Geometry: final body of the model. Coordinates: model frame, mm. Round coordinates to 2 decimals unless told otherwise and drop trailing zeros. Loops run counter-clockwise (first coordinate to the right, second up) from the corner with the lowest first, then second, coordinate; pieces in that order, holes last. Notation, with made-up numbers: (88, 22.5) - (139, 22.5) arc R19 ccw to (139, 46.5) - close; hole circle Ø7 at (54, 79.25). An arc over 180 degrees is marked (long way). Return JSON: item names as keys, results as strings. Group by question number.
1. Section A-A on x = -28. Return loops of the section in (y, z).
2. First-contact query: pin 1 Ø2 at (y, z) = (0, 0) entering from -X; pin 2 Ø3 at (x, z) = (8, -2) entering from -Y; pin 3 Ø1.5 at (x, y) = (-24, -2) entering from -Z; pin 4 Ø3.5 at (y, z) = (0, 0) entering from -X. Flat tips, straight axial feed; report the tip coordinate or a pass-through.
3. Material intervals for probe 1 along Y at (x, z) = (48.05, 0); probe 2 along Y at (x, z) = (-43, 0); probe 3 along Z at (x, y) = (-44.5, 0.5), sorted ascending.
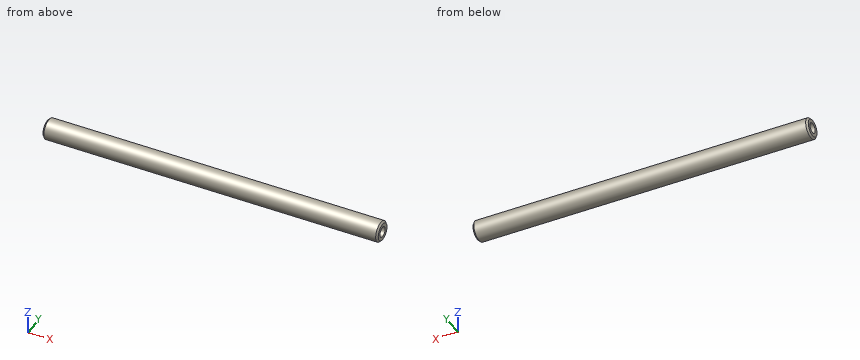
from build123d import *

# Parameters (mm, degrees)
SKETCH_1_W                     = 99
SKETCH_1_H                     = 3
CHAMFER_1_SIZE                 = 0.5
M3X0_5_1_D                     = 2.5
M3X0_5_1_DEPTH                 = 8.5
M3X0_5_1_CBORE_D               = 3
M3X0_5_1_CBORE_DEPTH           = 6
M3X0_5_1_TIP                   = 0.751075774
M3X0_5_1_ON_FACE_2_D           = 2.5
M3X0_5_1_ON_FACE_2_DEPTH       = 8.5
M3X0_5_1_ON_FACE_2_CBORE_D     = 3
M3X0_5_1_ON_FACE_2_CBORE_DEPTH = 6
M3X0_5_1_ON_FACE_2_TIP         = 0.751075774


with BuildPart() as part:
    # ｽｹｯﾁ1 → 回転1 (revolve)
    with BuildSketch(Plane.XY, mode=Mode.PRIVATE) as revolve_1_sk:
        with Locations((0, 1.5)):
            Rectangle(SKETCH_1_W, SKETCH_1_H)
    revolve(revolve_1_sk.sketch.rotate(Axis((0, 0, 0), (1, 0, 0)), 90), axis=Axis((0, 0, 0), (1, 0, 0)))

    # 面取り1
    chamfer_1_edges = [part.edges().sort_by_distance(p)[0] for p in [
        (49.5, 0, -3),
        (-49.5, 0, -3),
    ]]
    chamfer(chamfer_1_edges, length=CHAMFER_1_SIZE)

    # M3x0.5 ねじ穴1
    with Locations(Plane(origin=(49.5, 0, 0), x_dir=(0, 0, 1), z_dir=(1, 0, 0))):
        with Locations((0, 0)):
            CounterBoreHole(M3X0_5_1_D / 2, M3X0_5_1_CBORE_D / 2, M3X0_5_1_CBORE_DEPTH, depth=M3X0_5_1_DEPTH)
            with Locations((0, 0, -(M3X0_5_1_DEPTH + M3X0_5_1_TIP / 2))):  # 118° drill point
                Cone(0, M3X0_5_1_D / 2, M3X0_5_1_TIP, mode=Mode.SUBTRACT)

    # M3x0.5 ねじ穴1 on face 2
    with Locations(Plane(origin=(-49.5, 0, 0), x_dir=(0, 0, -1), z_dir=(-1, 0, 0))):
        with Locations((0, 0)):
            CounterBoreHole(M3X0_5_1_ON_FACE_2_D / 2, M3X0_5_1_ON_FACE_2_CBORE_D / 2, M3X0_5_1_ON_FACE_2_CBORE_DEPTH, depth=M3X0_5_1_ON_FACE_2_DEPTH)
            with Locations((0, 0, -(M3X0_5_1_ON_FACE_2_DEPTH + M3X0_5_1_ON_FACE_2_TIP / 2))):  # 118° drill point
                Cone(0, M3X0_5_1_ON_FACE_2_D / 2, M3X0_5_1_ON_FACE_2_TIP, mode=Mode.SUBTRACT)


solid = part.part
Taken from the geometry:
{
 "1": {"outline": "circle Ø6 at (0, 0)"},
 "2": {"pin 1": "x = -40.85", "pin 2": "y = -2.96", "pin 3": "z = -2.73", "pin 4": "x = -49.5"},
 "3": {"probe 1": "-3 to -1.5, 1.5 to 3", "probe 2": "-3 to -1.25, 1.25 to 3", "probe 3": "-2.96 to -1.41, 1.41 to 2.96"}
}
